```python
from build123d import *

# Parameters (mm, degrees)
SKETCH1_R           = 2.6
SKETCH1_R_2         = 2.2
SKETCH1_R_3         = 7.6
BOSS_EXTRUDE1_DEPTH = 1.8
FILLET1_R           = 3
FILLET2_R           = 1.4
SCALE1_SCALE        = 1.15


with BuildPart() as part:
    # Sketch1 → Boss-Extrude1 (new body)
    with BuildSketch(Plane(origin=(0, 0, 0), x_dir=(1, 0, 0), z_dir=(0, 1, 0))):
        Polygon((20.3, 35.160631394), (-20.3, 35.160631394), (-40.6, 0), (-20.3, -35.160631394), (20.3, -35.160631394), (40.6, 0), align=None)
        with Locations((-18.636201283, -32.21652123)):
            Circle(SKETCH1_R, mode=Mode.SUBTRACT)
        with Locations((18.582225165, -32.247684356)):
            Circle(SKETCH1_R, mode=Mode.SUBTRACT)
        with Locations((37.218426448, -0.031163126)):
            Circle(SKETCH1_R, mode=Mode.SUBTRACT)
        with Locations((-37.218426448, 0.031163126)):
            Circle(SKETCH1_R, mode=Mode.SUBTRACT)
        with BuildLine():
            Line((-32.142053523, 3.218057696), (-18.857946477, 26.226806032))
            Line((-18.857946477, 26.226806032), (-10.521325069, 11.78735419))
            ThreePointArc((-10.521325069, 11.78735419), (-13.68320138, 7.9), (-15.468810706, 3.218057696))
            Line((-15.468810706, 3.218057696), (-32.142053523, 3.218057696))
        make_face(mode=Mode.SUBTRACT)
        with BuildLine():
            Line((-18.857946477, -26.226806032), (-32.142053523, -3.218057696))
            Line((-32.142053523, -3.218057696), (-15.468810706, -3.218057696))
            ThreePointArc((-15.468810706, -3.218057696), (-13.68320138, -7.9), (-10.521325069, -11.78735419))
            Line((-10.521325069, -11.78735419), (-18.857946477, -26.226806032))
        make_face(mode=Mode.SUBTRACT)
        with BuildLine():
            Line((13.284107046, -29.444863729), (-13.284107046, -29.444863729))
            Line((-13.284107046, -29.444863729), (-4.947485637, -15.005411886))
            ThreePointArc((-4.947485637, -15.005411886), (0, -15.8), (4.947485637, -15.005411886))
            Line((4.947485637, -15.005411886), (13.284107046, -29.444863729))
        make_face(mode=Mode.SUBTRACT)
        with BuildLine():
            Line((32.142053523, -3.218057696), (18.857946477, -26.226806032))
            Line((18.857946477, -26.226806032), (10.521325069, -11.78735419))
            ThreePointArc((10.521325069, -11.78735419), (13.68320138, -7.9), (15.468810706, -3.218057696))
            Line((15.468810706, -3.218057696), (32.142053523, -3.218057696))
        make_face(mode=Mode.SUBTRACT)
        with BuildLine():
            Line((18.857946477, 26.226806032), (32.142053523, 3.218057696))
            Line((32.142053523, 3.218057696), (15.468810706, 3.218057696))
            ThreePointArc((15.468810706, 3.218057696), (13.68320138, 7.9), (10.521325069, 11.78735419))
            Line((10.521325069, 11.78735419), (18.857946477, 26.226806032))
        make_face(mode=Mode.SUBTRACT)
        with BuildLine():
            Line((-13.284107046, 29.444863729), (13.284107046, 29.444863729))
            Line((13.284107046, 29.444863729), (4.947485637, 15.005411886))
            ThreePointArc((4.947485637, 15.005411886), (0, 15.8), (-4.947485637, 15.005411886))
            Line((-4.947485637, 15.005411886), (-13.284107046, 29.444863729))
        make_face(mode=Mode.SUBTRACT)
        with Locations((-18.582225165, 32.247684356)):
            Circle(SKETCH1_R, mode=Mode.SUBTRACT)
        with Locations((18.636201283, 32.21652123)):
            Circle(SKETCH1_R, mode=Mode.SUBTRACT)
        with Locations((5.763168727, -9.982101048)):
            Circle(SKETCH1_R_2, mode=Mode.SUBTRACT)
        with Locations((-5.736740168, 9.936325441)):
            Circle(SKETCH1_R_2, mode=Mode.SUBTRACT)
        with Locations((0.052857117, 0)):
            Circle(SKETCH1_R_3, mode=Mode.SUBTRACT)
    extrude(amount=BOSS_EXTRUDE1_DEPTH)

    # Fillet1
    fillet1_edges = [part.edges().sort_by_distance(p)[0] for p in [
        (40.6, 0.9, 0),
        (20.3, 0.9, 35.160631394),
        (-20.3, 0.9, 35.160631394),
        (-40.6, 0.9, 0),
        (-20.3, 0.9, -35.160631394),
        (20.3, 0.9, -35.160631394),
    ]]
    fillet(fillet1_edges, radius=FILLET1_R)

    # Fillet2
    fillet2_edges = [part.edges().sort_by_distance(p)[0] for p in [
        (-32.142053523, 0.9, -3.218057696),
        (-15.468810706, 0.9, -3.218057696),
        (-10.521325069, 0.9, -11.78735419),
        (-18.857946477, 0.9, -26.226806032),
        (-18.857946477, 0.9, 26.226806032),
        (-10.521325069, 0.9, 11.78735419),
        (-15.468810706, 0.9, 3.218057696),
        (-32.142053523, 0.9, 3.218057696),
        (13.284107046, 0.9, 29.444863729),
        (4.947485637, 0.9, 15.005411886),
        (-4.947485637, 0.9, 15.005411886),
        (-13.284107046, 0.9, 29.444863729),
        (32.142053523, 0.9, 3.218057696),
        (15.468810706, 0.9, 3.218057696),
        (10.521325069, 0.9, 11.78735419),
        (18.857946477, 0.9, 26.226806032),
        (18.857946477, 0.9, -26.226806032),
        (10.521325069, 0.9, -11.78735419),
        (15.468810706, 0.9, -3.218057696),
        (32.142053523, 0.9, -3.218057696),
        (-13.284107046, 0.9, -29.444863729),
        (-4.947485637, 0.9, -15.005411886),
        (4.947485637, 0.9, -15.005411886),
        (13.284107046, 0.9, -29.444863729),
    ]]
    fillet(fillet2_edges, radius=FILLET2_R)


with BuildPart() as part_1:
    # Scale1: scaled about (-0.004144331, 0.9, -0.000288654)
    add(part.part.scale(SCALE1_SCALE).moved(Location((0.00062165, -0.135, 4.3298e-05))))


solid = part_1.part
```
Build history of the part. All positions in model axes, mm. A direction names the side the tool comes from. Give positions to 0.01 mm unless a question says otherwise; leave off trailing zeros. Order: outer loops, then holes, each group sorted by start corner. A loop starts at its lowest first (then second) coordinate and runs counter-clockwise, first axis right, second up. Notation, with made-up numbers: M 36.25,-33.75 L 59.25,-33.75 A20 cw 59.25,-10.75 Z; hole C 41.5,-38.5 d9. An arc over 180 degrees is marked long. Return JSON: item names as keys, results as strings.
Q1. 3-axis set-ups, long thin cutter, end or side, ignore diameter. For faces 1 (the face through (0, 1, -40.435)), 2 (the face through (-12.53, 0.91, -13.63)): which of +Z, -Z, +X, -X, +Y, -Y reach the whole face in a straight line?
Answer list:
{"face 1": "-Z, +X, -X, +Y, -Y", "face 2": "+Y, -Y"}
Q2. Two-plate mould, pull along X, no slides. Class faces 3 (the face through (-15.703, 0.886, -9.14)), 4 (the face through (23.1, 0.91, 39.96)), 5 (the face through (-23.1, 0.91, 39.96)): pulls with the +X half, pulls with the -X half, needs draft (parallel to the pull), parting line crosses it, or undercut.
Answer list:
{"face 3": "undercut", "face 4": "pulls with the +X half", "face 5": "pulls with the -X half"}
Q3. Flat gauge pins, fed straight in: pin 1 (4.5 mm diameter, centred on x = 6.63, z = 11.48, fed in from +Y); pin 2 (0.6 mm diameter, centred on x = -30.5, y = 1, fed in from +Z); pin 3 (0.6 mm diameter, centred on x = 27.5, y = 1, fed in from +Z); pin 4 (0.6 mm diameter, centred on x = 24.5, y = 1, fed in from -Z). Where does each tip first touch, or does it go through?
Answer list:
{"pin 1": "passes through", "pin 2": "stops at z = 28.56", "pin 3": "stops at z = 33.76", "pin 4": "stops at z = -38.93"}
Q4. Band-saw the part on B-B (z = -21). Give the cut face in (x, y) (3 decimals), then the cut area to 3 significant figures.
Answer list:
{"outline": "M -34.565,-0.135 L -26.975,-0.135 L -26.975,1.935 L -34.565,1.935 Z; M -16.397,-0.135 L -7.85,-0.135 L -7.85,1.935 L -16.397,1.935 Z; M 7.852,-0.135 L 16.398,-0.135 L 16.398,1.935 L 7.852,1.935 Z; M 26.976,-0.135 L 34.566,-0.135 L 34.566,1.935 L 26.976,1.935 Z", "area": "66.8 mm^2"}
Q5. Band-saw the part on A-A (x = 33). Give the cut face in (y, z) (3 decimals).
Answer list:
{"outline": "M -0.135,-23.713 L 1.935,-23.713 L 1.935,-10.567 L -0.135,-10.567 Z; M -0.135,-3.701 L 1.935,-3.701 L 1.935,3.701 L -0.135,3.701 Z; M -0.135,10.567 L 1.935,10.567 L 1.935,23.713 L -0.135,23.713 Z"}
Q6. Band-saw the part on C-C (y = 1). Count the separate pieces of the cut face and the enclosed holes in it, then the cut area to 3 significant figures.
Answer list:
{"separate pieces": "1", "enclosed holes": "15", "area": "3,190 mm^2"}
Q7. Band-saw the part on D-D (x = -37). Give the cut face in (y, z) (3 decimals), then the cut area to 3 significant figures.
Answer list:
{"outline": "M -0.135,-16.782 L 1.935,-16.782 L 1.935,16.783 L -0.135,16.783 Z", "area": "69.5 mm^2"}
Q8. Wall check: probe 1 along Z at (x, y) = (-21.5, 1.5); probe 2 along Z at (x, y) = (0, 0.35); probe 3 along X at (y, z) = (1.1, 5). Give the ranges that are in metal, low to high. Write a range as from..to.
Answer list:
{"probe 1": "z = -40.43..-40.07, -34.1..-28.54, -3.7..3.7, 28.54..34.06, 40.04..40.43", "probe 2": "z = -40.43..-33.86, -18.17..-8.74, 8.74..18.17, 33.86..40.43", "probe 3": "x = -43.8..-35.75, -17.47..-7.11, 7.23..17.47, 35.76..43.8"}
